Drawing for the job (mm, zero at the part's lowest x, y, z). A direction names the side the tool comes from. Coordinates: 2 decimals unless noted, no trailing zeros. Loops run counter-clockwise (first coordinate to the right, second up) from the corner with the lowest first, then second, coordinate; pieces in that order, holes last. Notation, with made-up numbers: (43.25, 18) - (47.25, 18) arc R11 ccw to (47.25, 35) - close; hole circle Ø8 at (-17, 36). An arc over 180 degrees is marked (long way). Put each result on its own line as item: value.
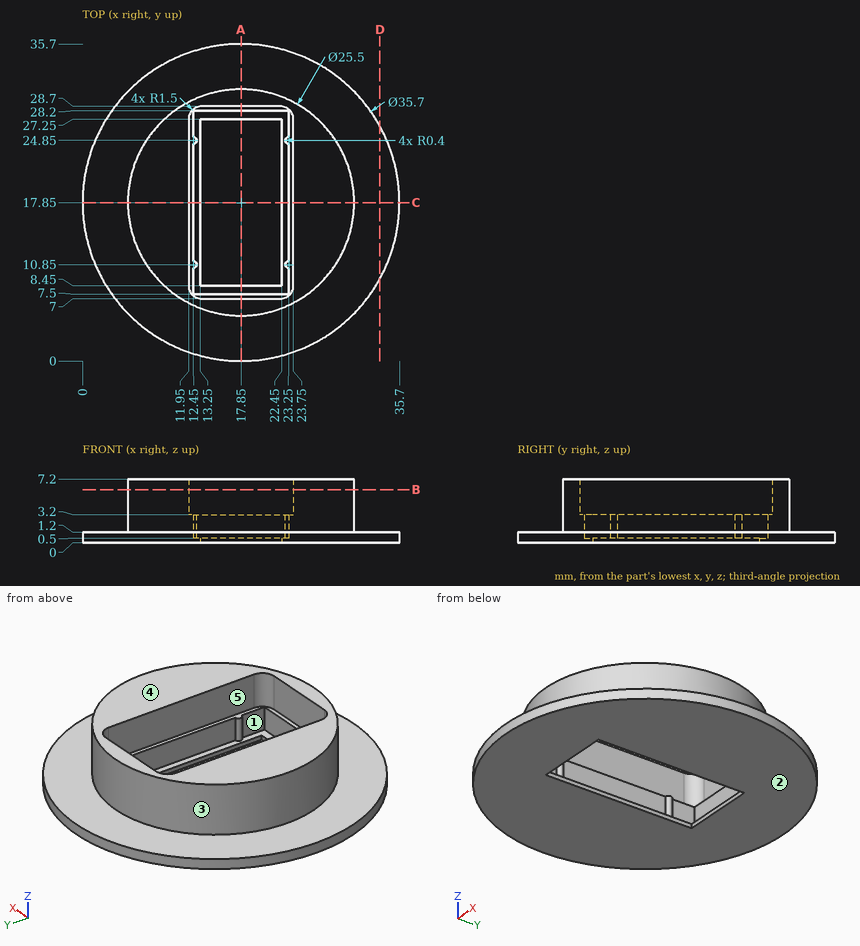
Q1. Mould opens along Y. For the marked faces 1, 2 and 3 say: +Y half, -Y half, draft (parallel to the pull), parting line (faces both ways), or undercut.
Determined:
face 1: undercut
face 2: draft
face 3: parting line
Q2. Slice it at B-B, the plane z = 6. Give the cut face in (x, y).
Determined:
outline: circle Ø25.5 at (17.85, 17.85); hole (11.95, 8.5) arc R1.5 ccw to (13.45, 7) - (22.25, 7) arc R1.5 ccw to (23.75, 8.5) - (23.75, 27.2) arc R1.5 ccw to (22.25, 28.7) - (13.45, 28.7) arc R1.5 ccw to (11.95, 27.2) - close
Q3. Slice it at D-D, the plane x = 33.5. Give the cut face in (y, z), then the cut area to 3 significant figures.
Determined:
outline: (9.27, 0) - (26.43, 0) - (26.43, 1.2) - (9.27, 1.2) - close
area: 20.6 mm2
Q4. Tool access for the marked faces 4 and 5: list every direction of +Z, -Z, +X, -X, +Y, -Y with a clear straight run to the whole face (end or side of a thin tool).
Determined:
face 4: +Z, +X, -X, +Y, -Y
face 5: +Z
Q5. Slice it at C-C, the plane y = 17.85. Give the cut face in (x, z), then the cut area to 3 significant figures.
Determined:
outline: (0, 0) - (13.25, 0) - (13.25, 0.5) - (12.45, 0.5) - (12.45, 3.2) - (11.95, 3.2) - (11.95, 7.2) - (5.1, 7.2) - (5.1, 1.2) - (0, 1.2) - close; (22.45, 0) - (35.7, 0) - (35.7, 1.2) - (30.6, 1.2) - (30.6, 7.2) - (23.75, 7.2) - (23.75, 3.2) - (23.25, 3.2) - (23.25, 0.5) - (22.45, 0.5) - close
area: 115 mm2
Q6. Wall check: L1, parallel to Z at x = 7.5, y = 7; L2, parallel to Y at x = 20, z = 1.75; L3, parallel to X at y = 19.5, z = 2.25. Give the ranges that are in metal, low to high. Write a range as from..to.
Determined:
L1: 0..1.2
L2: 5.28..7.5, 28.2..30.42
L3: 5.21..12.45, 23.25..30.49
Q7. Pin check, flat tips, straight feed: pin 1 Ø0.8 at (y, z) = (19, 1.5) entering from +X; pin 2 Ø3 at (x, z) = (8, 3) entering from -Y; pin 3 Ø3 at (y, z) = (26.5, 1.5) entering from +X; pin 4 Ø3.5 at (x, y) = (16.5, 22) entering from +Z. Stop position of each tip, or through.
Determined:
pin 1: x = 35.68
pin 2: y = 8.21
pin 3: x = 34.19
pin 4: through
Q8. Slice it at A-A, the plane x = 17.85. Give the cut face in (y, z), then the cut area to 4 significant figures.
Determined:
outline: (0, 0) - (8.45, 0) - (8.45, 0.5) - (7.5, 0.5) - (7.5, 3.2) - (7, 3.2) - (7, 7.2) - (5.1, 7.2) - (5.1, 1.2) - (0, 1.2) - close; (27.25, 0) - (35.7, 0) - (35.7, 1.2) - (30.6, 1.2) - (30.6, 7.2) - (28.7, 7.2) - (28.7, 3.2) - (28.2, 3.2) - (28.2, 0.5) - (27.25, 0.5) - close
area: 43.75 mm2
